from build123d import *

# Parameters (mm, degrees)
F1_DEPTH = 6.35
F2_R     = 2.9021462782
F3_DEPTH = 12.7


# Not quite as in the source:
# - a feature names something its author has since deleted; it is built from what else it names


with BuildPart() as f1:
    # F0 (on Top) → F1 (new body)
    with BuildSketch(Plane.XY):
        with BuildLine():
            Line((16.4344385917, 34.3732341826), (21.0574541174, 51.5500892249))
            Line((21.0574541174, 51.5500892249), (11.8116865515, 36.2228389391))
            ThreePointArc((11.8116865515, 36.2228389391), (-36.1240313077, 12.1105062684), (-12.4084995786, -36.0227586146))
            Line((-12.4084995786, -36.0227586146), (-16.8951376196, -48.5777822575))
            Line((-16.8951376196, -48.5777822575), (-8.5923329011, -37.1184834727))
            ThreePointArc((-8.5923329011, -37.1184834727), (35.960270838, -12.5884439569), (16.4344385917, 34.3732341826))
        make_face()
        with BuildLine():
            Line((-5.9558603501, -18.8854594723), (-10.1813612864, -30.1025640222))
            ThreePointArc((-10.1813612864, -30.1025640222), (-27.192206018, 8.287747581), (8.3393088452, 30.6639920157))
            Line((8.3393088452, 30.6639920157), (-8.4871153459, 2.7698433524))
            Line((-8.4871153459, 2.7698433524), (-0.5399501962, 5.5430036832))
            Line((-0.5399501962, 5.5430036832), (-12.3529230131, -20.1834143903))
            Line((-12.3529230131, -20.1834143903), (-5.9558603501, -18.8854594723))
        make_face(mode=Mode.SUBTRACT)
        with BuildLine():
            Line((10.5646807305, 0), (18.2668235735, 23.0856431528))
            Line((18.2668235735, 23.0856431528), (10.5646807305, 21.522889322))
            Line((10.5646807305, 21.522889322), (14.302094467, 29.2579978704))
            ThreePointArc((14.302094467, 29.2579978704), (28.7040765344, -9.3712062036), (-5.9558603501, -31.6943168745))
            Line((-5.9558603501, -31.6943168745), (16.3907865629, 1.182108589))
            Line((16.3907865629, 1.182108589), (10.5646807305, 0))
        make_face(mode=Mode.SUBTRACT)
    extrude(amount=F1_DEPTH)

    # F2 (on face) → F3 (cut)
    with BuildSketch(Plane.XY.offset(6.35)):
        with Locations((0, 34.4884768128)):
            Circle(F2_R)
    extrude(amount=-F3_DEPTH, mode=Mode.SUBTRACT)


solid = f1.part
For this review, take the finished solid that the model builds, in its own axes (mm). A direction names the side the tool comes from. Round coordinates to 2 decimals unless told otherwise and drop trailing zeros. Loops run counter-clockwise (first coordinate to the right, second up) from the corner with the lowest first, then second, coordinate; pieces in that order, holes last. Notation, with made-up numbers: (-37.75, -4) - (-1.75, -4) arc R30 cw to (-1.75, 22) - close; hole circle Ø8 at (65, 45.25). An arc over 180 degrees is marked (long way). Put each result on its own line as item: value. Start each with the question number.
1. Consider section C-C on y = -16. State the section outline as (x, z) points.
2. For faces 1 (the flat face through (13.52, 0.6, 3.13)), 2 (the flat face through (-14.62, -42.21, 3.13)), 3 (the flat face through (18.714, 42.841, 3.131)), list the 3-axis set-ups (+Z, -Z, +X, -X, +Y, -Y) from which the entire face can be reached by the end or side of a thin tool; tool diameter is ignored.
3. Consider section D-D on x = -30. State the section outline as (y, z) points, plus the area to 3 significant figures.
4. For probe 1 along Y at (x, z) = (0, 3.5); probe 2 along Y at (x, z) = (2.5, 1.75); probe 3 along X at (y, z) = (12, 1), list the stretches that pass through material, from the lowest coordinate up. Write a range as [from, to].
5. Consider section A-A on y = 9. State the section outline as (x, z) points, plus the area to 3 significant figures.
6. Mouldability with a two-part tool opening along Y and no side actions: class faces 4 (the cylindrical face through (28.895, -8.777, 3.131)), 5 (the flat face through (3, 5, 0)), 6 (the flat face through (-12.802, -42.928, 3.131)) as +Y half, -Y half, draft (parallel to the pull), parting line (faces both ways), or undercut.
7. Insertion check: P1, Ø5, axis at x = -25, y = -34.5, coming from the -Z side; P2, Ø3, axis at y = -34, z = 2.5, coming from the -X side. Each pin has a flat end and moves straight along its axis. Give the tip position at first contact, or say it passes through.
Result sheet:
1. outline: (-34.58, 0) - (-24.9, 0) - (-24.9, 6.35) - (-34.58, 6.35) - close; (-10.43, 0) - (4.71, 0) - (4.71, 6.35) - (-10.43, 6.35) - close; (25.65, 0) - (34.58, 0) - (34.58, 6.35) - (25.65, 6.35) - close
2. face 1: +Z, -Z
2. face 2: +Z, -Z, -X
2. face 3: +Z, -Z, +X
3. outline: (-23.49, 0) - (23.49, 0) - (23.49, 6.35) - (-23.49, 6.35) - close
3. area: 298 mm^2
4. probe 1: [-38.1, -31.78], [-22.93, 16.84], [30.84, 31.59], [37.39, 38.1]
4. probe 2: [-38.02, -31.5], [-19.25, 20.98], [31.01, 33.01], [35.96, 38.02]
4. probe 3: [-36.16, -25.81], [-2.92, 14.57], [28.49, 36.16]
5. outline: (-37.02, 0) - (-26.97, 0) - (-26.97, 6.35) - (-37.02, 6.35) - close; (-4.73, 0) - (13.57, 0) - (13.57, 6.35) - (-4.73, 6.35) - close; (29.39, 0) - (37.02, 0) - (37.02, 6.35) - (29.39, 6.35) - close
5. area: 228 mm^2
6. face 4: undercut
6. face 5: draft
6. face 6: -Y half
7. P1: through
7. P2: x = -19.88
